from build123d import *

# Parameters (mm, degrees)
F1_DEPTH = 63.5
F0_W     = 25.4
F0_H     = 19.05
F2_DEPTH = 25.4
F4_DEPTH = 10.16


with BuildPart() as f1:
    # F0 (on Front) → F1 (new body, symmetric)
    with BuildSketch(Plane.XZ):
        Polygon((22.225, 9.525), (-41.275, 9.525), (-41.275, -9.525), (41.275, -9.525), (41.275, 9.525), align=None)
    extrude(amount=F1_DEPTH, both=True)

    # F0 (on Front) → F2 (join, symmetric)
    with BuildSketch(Plane.XZ):
        with Locations((73.025, 52.4002)):
            Rectangle(F0_W, F0_H)
        with BuildLine():
            Line((22.225, 27.0002), (22.225, 9.525))
            Line((22.225, 9.525), (41.275, 9.525))
            Line((41.275, 9.525), (41.275, 27.0002))
            ThreePointArc((41.275, 27.0002), (45.9246798487, 38.2255201513), (57.15, 42.8752))
            Line((57.15, 42.8752), (60.325, 42.8752))
            Line((60.325, 42.8752), (60.325, 61.9252))
            Line((60.325, 61.9252), (57.15, 61.9252))
            ThreePointArc((57.15, 61.9252), (57.9844058032, 61.9152310319), (58.8183352619, 61.8853298185))
            add(Edge.make_bspline(
                [(53.4926140261, 61.7331692488), (55.2678452384, 61.7956996578), (57.0438857135, 61.8460829523), (58.8183352619, 61.8853298185)],
                knots=[108.9494313883, 108.9494313883, 108.9494313883, 108.9494313883, 112.9614089083, 112.9614089083, 112.9614089083, 112.9614089083], degree=3))
            ThreePointArc((53.4926140261, 61.7331692488), (31.1934032456, 50.3670720613), (22.225, 27.0002))
        make_face()
    extrude(amount=F2_DEPTH, both=True)

    # F0 (on Front) → F3 (revolve)
    with BuildSketch(Plane.XZ):
        Polygon((85.725, 66.675), (85.725, 61.9252), (85.725, 42.8752), (85.725, 38.1), (111.125, 38.1), (111.125, 66.675), align=None)
    revolve(axis=Axis((85.725, 0, 52.3875), (0, 0, -1)))

    # F0 (on Front) → F4 (join, symmetric)
    with BuildSketch(Plane.XZ):
        with BuildLine():
            add(Edge.make_bspline(
                [(-41.275, 9.525), (-42.3271025426, 49.3791151261), (5.2843600658, 60.0350908151), (53.4926140261, 61.7331692488)],
                knots=[0, 0, 0, 0, 108.9494313883, 108.9494313883, 108.9494313883, 108.9494313883], degree=3))
            Line((-41.275, 9.525), (22.225, 9.525))
            Line((22.225, 9.525), (22.225, 27.0002))
            ThreePointArc((22.225, 27.0002), (31.1934032456, 50.3670720613), (53.4926140261, 61.7331692488))
        make_face()
    extrude(amount=F4_DEPTH, both=True)


solid = f1.part
Read the model definition and answer for the solid it produces. Units are mm, in the model's axes. A direction names the side the tool comes from. Give positions to 0.01 mm unless a question says otherwise; leave off trailing zeros. Write each loop counter-clockwise with the first axis right and the second up, starting at its lowest first coordinate (ties: lowest second). Pieces come first, ordered by that corner, then holes. Notation, with made-up numbers: M 6.5,87 L 57.5,87 A32 ccw 57.5,113 Z; hole C -15,21 d11. An arc over 180 degrees is marked long. One line per item, written item: value. Start each with the question number.
(1) A tool of negligible diameter and unlimited length cuts with its end or side. For faces 4 (the flat face through (41.275, -1, 4)), 5 (the flat face through (60, 2, 42.875)), 6 (the flat face through (22.225, -18, 18)), 7 (the cylindrical face through (31.43, 17.67, 50.63)), 8 (the flat face through (60, -2, 61.925)), from which of +Z, -Z, +X, -X, +Y, -Y can it reach the whole face along a straight path? Write none if from no direction.
(2) Find the intervals of material crossed by line 1 (Z direction, x = -9.5, y = -53) (3 decimals); line 2 (X direction, y = -11.5, z = 28); line 3 (Y direction, x = -16, z = 47), in increasing order.
(3) Flat-ended cylindrical pins translate along their axes: pin 1 Ø17 at (y, z) = (15, 15) entering from -X; pin 2 Ø1.5 at (x, z) = (-14, 21) entering from +Y; pin 3 Ø8 at (y, z) = (-21.5, 26) entering from +X; pin 4 Ø2 at (y, z) = (15, -0.5) entering from +X (3 decimals). Find the tip coordinate at first contact, or state that the pin passes through.
(4) Find section B-B (x = 95). Determine the outline of the cut face in (y, z) (3 decimals), plus the area to 3 significant figures.
(5) Determine the mould class of faces 1 (the cylindrical face through (45.8, -0.4, 38.1)), 2 (the flat face through (86, 0, 38.1)), 3 (the cylindrical face through (31.43, -17.89, 50.63)) for opening direction X: pulls with the +X half, pulls with the -X half, needs draft (parallel to the pull), parting line crosses it, or undercut.
(6) Find section A-A (y = -38). Determine the outline of the cut face in (x, z) (3 decimals), plus the area to 3 significant figures.
Results below:
1. face 4: -Z, +X, +Y, -Y
1. face 5: -Z
1. face 6: +Z, -X, -Y
1. face 7: +Z, -X, +Y
1. face 8: +Z, -X
2. line 1: z = -9.525 to 9.525
2. line 2: x = 22.24 to 41.31
2. line 3: y = -10.16 to 10.16
3. pin 1: stops at x = -41.29
3. pin 2: stops at y = 10.16
3. pin 3: stops at x = 41.56
3. pin 4: stops at x = 41.275
4. outline: M -23.646,38.1 L 23.646,38.1 L 23.646,66.675 L -23.646,66.675 Z
4. area: 1,350 mm^2
5. face 1: undercut
5. face 2: needs draft
5. face 3: pulls with the -X half
6. outline: M -41.275,-9.525 L 41.275,-9.525 L 41.275,9.525 L -41.275,9.525 Z
6. area: 1,570 mm^2
